Design review of the part shown in the three views and the two pictorial views. Dimensions are in mm from the part's minimum x, y and z. A direction names the side the tool comes from. Give positions to 0.01 mm unless a question says otherwise; leave off trailing zeros. Order: outer loops, then holes, each group sorted by start corner. A loop starts at its lowest first (then second) coordinate and runs counter-clockwise, first axis right, second up.
Item 1: Consider section D-D (y = 8). Give the boundary of the cut face in (x, z).
Item 2: Consider section C-C (x = 86.5). Give the boundary of the cut face in (y, z) (3 decimals).
Item 3: The part is to be moulded in two halves that separate along Y. For the marked faces 1, 2, 3 and 4, say which applies: released by +Y, released by -Y, zero draft, split by the parting line, or undercut.
Item 4: Consider section B-B (y = 13). Give the boundary of the cut face in (x, z).
Item 5: Consider section A-A (z = 20). Give the boundary of the cut face in (x, y) (3 decimals), plus the area to 3 significant figures.
Item 6: For probe 1 along X at (y, z) = (24.5, 30.5); probe 2 along X at (y, z) = (21, 18); probe 3 along Y at (x, z) = (23.5, 4.5), list the stretches that pass through material, from the lowest coordinate up.
Item 7: Machinability: for the marked faces 5, 6, 7 and 8, which of the approach directions +Z, -Z, +X, -X, +Y, -Y give a long, thin tool a straight path to every point of the face, cutting with its end or side? Answer none if there is none.
Item 8: For P1, Ø4, axis at y = 21.5, z = 9.5, coming from the +X side; P2, Ø7.5, axis at y = 26.5, z = 18, coming from the +X side; P3, Ø1, axis at x = 60, y = 20.5, coming from the -Z side, all flat-tipped, find the tip position at first contact; note any pin that passes through.
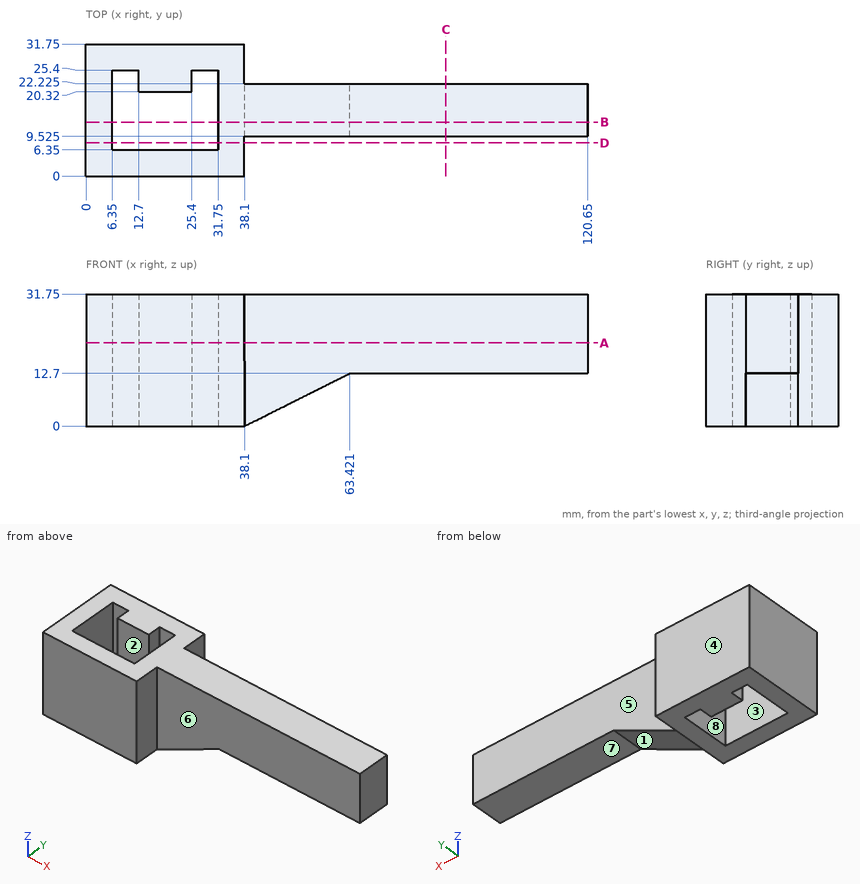
Resolved:
1. outline: (0, 0) - (6.35, 0) - (6.35, 31.75) - (0, 31.75) - close; (31.75, 0) - (38.1, 0) - (38.1, 31.75) - (31.75, 31.75) - close
2. outline: (9.525, 12.7) - (22.225, 12.7) - (22.225, 31.75) - (9.525, 31.75) - close
3. face 1: zero draft
3. face 2: undercut
3. face 3: undercut
3. face 4: released by +Y
4. outline: (0, 0) - (6.35, 0) - (6.35, 31.75) - (0, 31.75) - close; (31.75, 0) - (38.1, 0) - (63.42, 12.7) - (120.65, 12.7) - (120.65, 31.75) - (31.75, 31.75) - close
5. outline: (0, 0) - (38.1, 0) - (38.1, 9.525) - (120.65, 9.525) - (120.65, 22.225) - (38.1, 22.225) - (38.1, 31.75) - (0, 31.75) - close; hole (6.35, 6.35) - (31.75, 6.35) - (31.75, 25.4) - (25.4, 25.4) - (25.4, 20.32) - (12.7, 20.32) - (12.7, 25.4) - (6.35, 25.4) - close
5. area: 1,840 mm2
6. probe 1: x = 0 to 6.35, 12.7 to 25.4, 31.75 to 38.1
6. probe 2: x = 0 to 6.35, 12.7 to 25.4, 31.75 to 120.65
6. probe 3: y = 0 to 6.35, 20.32 to 31.75
7. face 5: +Z, -Z, +X, +Y
7. face 6: +Z, -Z, +X, -Y
7. face 7: -Z, +X, +Y, -Y
7. face 8: +Z, -Z
8. P1: stops at x = 61.03
8. P2: stops at x = 38.1
8. P3: stops at z = 10.73
